```python
from build123d import *

# Parameters (mm, degrees)
SKETCH1_W           = 127
SKETCH1_H           = 685.8
BOSS_EXTRUDE1_DEPTH = 25.4
BOSS_EXTRUDE2_DEPTH = 127
BOSS_EXTRUDE3_DEPTH = 685.8


with BuildPart() as part:
    # Sketch1 → Boss-Extrude1 (new body)
    with BuildSketch(Plane.XY):
        with Locations((-63.5, 342.9)):
            Rectangle(SKETCH1_W, SKETCH1_H)
    extrude(amount=BOSS_EXTRUDE1_DEPTH)

    # Sketch2 → Boss-Extrude2 (add)
    with BuildSketch(Plane.ZY.offset(127)):
        with BuildLine():
            Line((44.45, 514.35), (25.4, 514.35))
            Line((25.4, 514.35), (25.4, 476.25))
            Line((25.4, 476.25), (44.45, 476.25))
            ThreePointArc((44.45, 476.25), (63.5, 495.3), (44.45, 514.35))
        make_face()
        with BuildLine():
            Line((44.45, 209.55), (25.4, 209.55))
            Line((25.4, 209.55), (25.4, 171.45))
            Line((25.4, 171.45), (44.45, 171.45))
            ThreePointArc((44.45, 171.45), (63.5, 190.5), (44.45, 209.55))
        make_face()
    extrude(amount=-BOSS_EXTRUDE2_DEPTH)

    # Sketch3 → Boss-Extrude3 (add)
    with BuildSketch(Plane.XZ):
        with BuildLine():
            Line((-88.9, -25.4), (-88.9, 0))
            Line((-88.9, 0), (-38.1, 0))
            Line((-38.1, 0), (-38.1, -25.4))
            ThreePointArc((-38.1, -25.4), (-63.5, -50.8), (-88.9, -25.4))
        make_face()
    extrude(amount=-BOSS_EXTRUDE3_DEPTH)


solid = part.part
```
Here's how the part is built. I have some questions about the finished solid (model axes, mm). A direction names the side the tool comes from. Coordinates: 2 decimals unless noted, no trailing zeros. Order: outer loops, then holes, each group sorted by start corner. A loop starts at its lowest first (then second) coordinate and runs counter-clockwise, first axis right, second up. Notation, with made-up numbers: (82, 38) -> (104, 38) arc R21 ccw to (104, 45) -> close; hole circle Ø7 at (62, 83.5). An arc over 180 degrees is marked (long way). Return JSON: item names as keys, results as strings.
1) If I drill on probe 1 along Y at (x, z) = (-68.5, 30.5); probe 2 along Z at (x, y) = (-21, 355); probe 3 along Y at (x, z) = (-47.5, 45.5), over which ranges is the centre line in solid material (lowest first)?
Conclusion:
{"probe 1": "y = 171.45 to 209.55, 476.25 to 514.35", "probe 2": "z = 0 to 25.4", "probe 3": "y = 171.48 to 209.52, 476.28 to 514.32"}
2) If we section it at D-D on y = 615: List the corners of the cut face in (x, z) for me, plus the area to 3 significant figures.
Conclusion:
{"outline": "(-127, 0) -> (-88.9, 0) -> (-88.9, -25.4) arc R25.4 ccw to (-38.1, -25.4) -> (-38.1, 0) -> (0, 0) -> (0, 25.4) -> (-127, 25.4) -> close", "area": "5,530 mm²"}
3) I'm going to push flat-ended pins straight in: P1, Ø2, axis at x = -87, y = 315.5, coming from the +Z side; P2, Ø9.5, axis at x = -63.5, z = 38.5, coming from the +Y side; P3, Ø7.5, axis at y = 324.5, z = -11.5, coming from the -X side. Where does each tip first touch, or does it pass through?
Conclusion:
{"P1": "stops at z = 25.4", "P2": "stops at y = 514.35", "P3": "stops at x = -88.9"}
4) If we section it at C-C on z = -12: List the corners of the cut face in (x, y) for me, plus the area to 3 significant figures.
Conclusion:
{"outline": "(-88.9, 0) -> (-38.1, 0) -> (-38.1, 685.8) -> (-88.9, 685.8) -> close", "area": "34,800 mm²"}
5) If we section it at B-B on y = 495.3: List the corners of the cut face in (x, z) for me.
Conclusion:
{"outline": "(-127, 0) -> (-88.9, 0) -> (-88.9, -25.4) arc R25.4 ccw to (-38.1, -25.4) -> (-38.1, 0) -> (0, 0) -> (0, 63.5) -> (-127, 63.5) -> close"}
6) Thinking about a two-plate mould opening in Y: for faces 1 (the flat face through (-64, 685.8, -5)), 2 (the flat face through (-64, 476.25, 35)), 3 (the flat face through (0, 338, 17)), which applies, +Y half, -Y half, draft (parallel to the pull), parting line (faces both ways), or undercut?
Conclusion:
{"face 1": "+Y half", "face 2": "undercut", "face 3": "draft"}
7) On a 3-axis mill with a long thin cutter (end or side, diameter ignored), from which of +Z, -Z, +X, -X, +Y, -Y can I reach the whole of each face in a straight line? I mean faces 4 (the flat face through (-64, 209.55, 35)), 5 (the flat face through (-64, 171.45, 35)), 6 (the flat face through (-38.1, 338, -13)), 7 (the flat face through (-64, 514.35, 35)). Say none if no direction works.
Conclusion:
{"face 4": "+Z, +X, -X", "face 5": "+Z, +X, -X, -Y", "face 6": "-Z, +X, +Y, -Y", "face 7": "+Z, +X, -X, +Y"}
8) If we section it at A-A on x = -110: List the corners of the cut face in (y, z) for me.
Conclusion:
{"outline": "(0, 0) -> (685.8, 0) -> (685.8, 25.4) -> (514.35, 25.4) -> (514.35, 44.45) arc R19.05 ccw to (476.25, 44.45) -> (476.25, 25.4) -> (209.55, 25.4) -> (209.55, 44.45) arc R19.05 ccw to (171.45, 44.45) -> (171.45, 25.4) -> (0, 25.4) -> close"}
